Verification items for the finished model (mm, model axes). A direction names the side the tool comes from. Coordinates: 2 decimals unless noted, no trailing zeros. Order: outer loops, then holes, each group sorted by start corner. A loop starts at its lowest first (then second) coordinate and runs counter-clockwise, first axis right, second up. Notation, with made-up numbers: M -19.5,11 L 23.5,11 A13 ccw 23.5,19 Z; hole C -4.5,61 d7. An arc over 180 degrees is marked long. Return JSON: item names as keys, results as strings. Group by question number.
1. Section check A-A, the plane y = 30. Record the cut outline in (x, z).
2. Gauge pin test, flat ends, axial feed: pin 1 (11 mm diameter, centred on x = -2, y = 23.5, fed in from +Z); pin 2 (6 mm diameter, centred on x = 1, z = 8.5, fed in from +Y); pin 3 (4.5 mm diameter, centred on y = 10, z = -4.5, fed in from -X); pin 4 (8 mm diameter, centred on y = 19.5, z = 5.5, fed in from +X). Record the tip position at first contact, or that the pin passes through.
3. Mould release check, pull along Z, two halves, no side actions. Record for faces 1 (the cylindrical face through (-10.95, 1.01, -10.5)), 2 (the flat face through (0, 0, 0)), 3 (the cylindrical face through (-6.55, 26.4, -7.02)), 4 (the conical face through (-7.361, 33.873, -3.086)): +Z half, -Z half, draft (parallel to the pull), parting line (faces both ways), or undercut.
4. Section check D-D, the plane x = 10.25. Record the cut outline in (y, z), plus the area to 3 significant figures.
5. Section check B-B, the plane y = 12.5. Record the cut outline in (x, z), plus the area to 3 significant figures.
6. Section check C-C, the plane z = 7.5. Record the cut outline in (x, y), plus the area to 3 significant figures.
7. Material ranges on line 1 along X through (y, z) = (26.75, -6.75); line 2 along Z through (x, y) = (-4.5, 29); line 3 along Z through (x, y) = (2.25, 14.5), recorded low to high.
8. Set-up check for faces 5 (the flat face through (-8.5, 14, -6)), 6 (the cylindrical face through (7.45, 21.3, -3)), 7 (the flat face through (-10, 7, 6)), 8 (the cylindrical face through (9.155, 4.482, -0.461)): record each of +Z, -Z, +X, -X, +Y, -Y from which the full face is reachable in a straight line by a thin tool's end or side.
Autodesk Inventor part; units mm, degrees
ref_plane "YZ Plane" through (0, 0, 0) normal (1, 0, 0) x (0, 1, 0)
ref_plane "XZ Plane" through (0, 0, 0) normal (0, 1, 0) x (-1, 0, 0)
ref_plane "XY Plane" through (0, 0, 0) normal (0, 0, 1) x (1, 0, 0)
sketch "Base Outline" plane through (0, 0, 0) normal (0, 1, 0) x (-1, 0, 0)
  line L0 (12, -11.5) -> (-12, -11.5)
  line L1 (-12, -11.5) -> (-12, 11.5)
  line L2 (-12, 11.5) -> (12, 11.5)
  line L3 (12, 11.5) -> (12, -11.5)
  point P0 (0, 0)
  dimension "d0" = 23
  dimension "d1" = 11.5
  dimension "d2" = 24
  dimension "d3" = 12
extrude "Base" add sketch "Base Outline" along normal blind 8.5
sketch "Pillar Outline" plane through (0, 8.5, 0) normal (0, 1, 0) x (1, 0, 0)
  line L0 (-8.5, 11.5) -> (8.5, 11.5)
  line L1 (8.5, 11.5) -> (8.5, 2)
  line L2 (8.5, 2) -> (-8.5, 2)
  line L3 (-8.5, 2) -> (-8.5, 11.5)
  line L4 (12, 11.5) -> (-12, 11.5)
  point P0 (0, 0)
  dimension "d6" = 0
  dimension "d7" = 9.5
  dimension "d8" = 17
  dimension "d9" = 8.5
extrude "Pillar" add sketch "Pillar Outline" along normal blind 25.5
sketch "Base Cutouts Outline" plane through (0, 8.5, 0) normal (0, 1, 0) x (1, 0, 0)
  line L0 (-8.5, -1) -> (-12, -1)
  line L1 (-12, -1) -> (-12, 11.5)
  line L2 (-12, 11.5) -> (-8.5, 11.5)
  line L3 (-8.5, 11.5) -> (-8.5, -1)
  line L4 (8.5, -1) -> (12, -1)
  line L5 (12, -1) -> (12, 11.5)
  line L6 (12, 11.5) -> (8.5, 11.5)
  line L7 (8.5, 11.5) -> (8.5, -1)
  line L8 (-8.5, 11.5) -> (-12, 11.5)
  line L9 (-12, 11.5) -> (-12, -11.5)
  line L10 (-8.5, 11.5) -> (-8.5, 2)
  line L11 (8.5, 2) -> (8.5, 11.5)
  line L12 (12, 11.5) -> (8.5, 11.5)
  line L13 (12, -11.5) -> (12, 11.5)
  point P0 (0, 0)
  dimension "d12" = 0
  dimension "d13" = 0
  dimension "d14" = 0
  dimension "d15" = 12.5
  dimension "d16" = 0
  dimension "d17" = 0
  dimension "d18" = 0
  dimension "d19" = 12.5
extrude "Base Cutouts" cut sketch "Base Cutouts Outline" against normal blind 6.5
sketch "Hole Positions" plane through (0, 34, 0) normal (0, 1, 0) x (1, 0, 0)
  line L0 (8.5, 11.5) -> (-8.5, 11.5)
  point P0 (0, 0)
  point P1 (4.5, 6.75)
  point P2 (-4.5, 6.75)
  dimension "d22" = 4.75
  dimension "d23" = 4.5
  dimension "d24" = 4.5
  dimension "d25" = 4.75
hole "Holes" at (4.5, 34, -6.75) at (-4.5, 34, -6.75) direction (0, -1, 0) diameter 4.134 depth 15 tip angle 118
chamfer "Base Chamfer" distance 3.5 angle 45 2 edges at (-12, 8.5, 6.25) (12, 8.5, 6.25)
fillet "Pillar Fillet" radius 3.5 10 edges at (-12, 1, -11.5) (-8.5, 18, -11.5) (-8.5, 21.25, -2) (8.5, 21.25, -2) (-8.5, 5.25, 1) (-12, 2.5, 11.5) (12, 2.5, 11.5) (8.5, 5.25, 1) (12, 1, -11.5) (8.5, 18, -11.5)
chamfer "Pillar Chamfer" distance 0.25 angle 45 8 edges at (-7.4749, 34, -3.0251) (-8.5, 34, -6.75) (-7.4749, 34, -10.4749) (0, 34, -11.5) (7.4749, 34, -10.4749) (8.5, 34, -6.75) (7.4749, 34, -3.0251) (0, 34, -2)
equation "\"d19\" = d15"
properties part number "LR Rail" material "Aluminum 6061"
Answers follow:
{
 "1": {"outline": "M -8.5,-8 A3.5 ccw -5,-11.5 L 5,-11.5 A3.5 ccw 8.5,-8 L 8.5,-5.5 A3.5 ccw 5,-2 L -5,-2 A3.5 ccw -8.5,-5.5 Z; hole C -4.5,-6.75 d4.13; hole C 4.5,-6.75 d4.13"},
 "2": {"pin 1": "z = -2", "pin 2": "y = 8.5", "pin 3": "x = -8.5", "pin 4": "through"},
 "3": {"face 1": "-Z half", "face 2": "draft", "face 3": "undercut", "face 4": "+Z half"},
 "4": {"outline": "M 0,-11.03 L 2,-11.03 L 2,0.53 L 6.75,0.53 L 6.75,11.03 L 0,11.03 Z", "area": "94.0 mm^2"},
 "5": {"outline": "M -8.5,-8 A3.5 ccw -5,-11.5 L 5,-11.5 A3.5 ccw 8.5,-8 L 8.5,-5.5 A3.5 ccw 5,-2 L -5,-2 A3.5 ccw -8.5,-5.5 Z", "area": "151 mm^2"},
 "6": {"outline": "M -12,0 L 12,0 L 12,5 L 8.5,8.5 L -8.5,8.5 L -12,5 Z", "area": "192 mm^2"},
 "7": {"line 1": "-8.5 to -6.57, -2.43 to 2.43, 6.57 to 8.5", "line 2": "-11.5 to -8.82, -4.68 to -2", "line 3": "-11.5 to -2"},
 "8": {"face 5": "-Z, -X, +Y", "face 6": "+Z, +X, +Y", "face 7": "+Z, -Z, -X, +Y", "face 8": "-Z, +X, +Y"}
}
